from build123d import *

# Parameters (mm, degrees)
BOSS_EXTRUDE1_DEPTH  = 10
SKETCH2_R            = 3
CUT_EXTRUDE1_DEPTH   = 10
LPATTERN1_COUNT      = 6
LPATTERN1_PITCH      = 10
LPATTERN1_COUNT_DIR2 = 4
LPATTERN1_PITCH_DIR2 = 10


with BuildPart() as part:
    # Sketch1 → Boss-Extrude1 (new body)
    with BuildSketch(Plane.XY):
        Polygon((0, 0), (0, 43.65799141), (40.804527919, 43.65799141), (40.804527919, 26.346979566), (67.056392035, 26.346979566), (67.056392035, 4.280195236), (67.056392035, 0), align=None)
    extrude(amount=BOSS_EXTRUDE1_DEPTH)

    # Sketch2 → Cut-Extrude1 (cut)
    with BuildSketch(Plane.XY.offset(10)):
        with Locations((6, 6)):
            Circle(SKETCH2_R)
    cut_extrude1 = extrude(amount=-CUT_EXTRUDE1_DEPTH, mode=Mode.SUBTRACT)

    # LPattern1: Cut-Extrude1 6 × 4, 4 skipped
    with Locations(*[(i * LPATTERN1_PITCH, j * LPATTERN1_PITCH_DIR2, 0) for i in range(LPATTERN1_COUNT) for j in range(LPATTERN1_COUNT_DIR2) if (i, j) not in ((0, 0), (4, 2), (4, 3), (5, 2), (5, 3))]):
        add(cut_extrude1, mode=Mode.SUBTRACT)


solid = part.part
The model under review builds one solid part; all positions refer to its coordinate system, in mm. Round coordinates to 2 decimals unless told otherwise and drop trailing zeros. Write each loop counter-clockwise with the first axis right and the second up, starting at its lowest first coordinate (ties: lowest second). Pieces come first, ordered by that corner, then holes. Notation, with made-up numbers: M -36.75,63.5 L 2.25,63.5 A27 ccw 2.25,89.5 Z; hole C 89,48.25 d9. An arc over 180 degrees is marked long. Answer as CSV lines item,"result". Start each with the question number.
Q1. The part is to be moulded in two halves that separate along X. For faces 1 (the face through (34, 0, 5)), 2 (the face through (23.6, 4.2, 5.1)), 3 (the face through (0, 22, 5)), say which applies: +X half, -X half, draft (parallel to the pull), parting line (faces both ways), or undercut.
Q2. Clearance check with a flat-ended pin moving along its axis: P1, Ø2, axis at y = 29, z = 2, coming from the +X side. State where the tip first meets the part, or that it passes through.
Q3. Consider section C-C, the plane z = 8.5. State how many separate pieces and enclosed holes the cut face has, then the cut area to 3 significant figures.
Q4. Consider section B-B, the plane y = 36. Give the boundary of the cut face in (x, z), then the cut area to 3 significant figures.
Q5. Consider section D-D, the plane x = 46. Give the boundary of the cut face in (y, z), then the cut area to 3 significant figures.
Q6. Consider section A-A, the plane x = 16. Give the boundary of the cut face in (y, z).
Q7. Wall thickness on line 1 along Y through (x, z) = (36, 5.5); line 2 along Y through (x, z) = (46, 7.5); line 3 along Y through (x, z) = (34.5, 2.5): over which ranges is each line inside the solid? List them lowest first.
Result set:
1,face 1,"draft"
1,face 2,"undercut"
1,face 3,"-X half"
2,P1,"stops at x = 40.8"
3,separate pieces,"1"
3,enclosed holes,"20"
3,area,"1,910 mm²"
4,outline,"M 0,0 L 3,0 L 3,10 L 0,10 Z; M 9,0 L 13,0 L 13,10 L 9,10 Z; M 19,0 L 23,0 L 23,10 L 19,10 Z; M 29,0 L 33,0 L 33,10 L 29,10 Z; M 39,0 L 40.8,0 L 40.8,10 L 39,10 Z"
4,area,"168 mm²"
5,outline,"M 0,0 L 3,0 L 3,10 L 0,10 Z; M 9,0 L 13,0 L 13,10 L 9,10 Z; M 19,0 L 26.35,0 L 26.35,10 L 19,10 Z"
5,area,"143 mm²"
6,outline,"M 0,0 L 3,0 L 3,10 L 0,10 Z; M 9,0 L 13,0 L 13,10 L 9,10 Z; M 19,0 L 23,0 L 23,10 L 19,10 Z; M 29,0 L 33,0 L 33,10 L 29,10 Z; M 39,0 L 43.66,0 L 43.66,10 L 39,10 Z"
7,line 1,"y = 0 to 3, 9 to 13, 19 to 23, 29 to 33, 39 to 43.66"
7,line 2,"y = 0 to 3, 9 to 13, 19 to 26.35"
7,line 3,"y = 0 to 3.4, 8.6 to 13.4, 18.6 to 23.4, 28.6 to 33.4, 38.6 to 43.66"
